Design review of the part built by this model. Coordinates are the model's own, in mm. Face numbers are marked on the shaded views. A direction names the side the tool comes from. Coordinates: 2 decimals unless noted, no trailing zeros. Order: outer loops, then holes, each group sorted by start corner. A loop starts at its lowest first (then second) coordinate and runs counter-clockwise, first axis right, second up. Notation, with made-up numbers: M 73.5,9.25 L 111.5,9.25 A19 ccw 111.5,20.25 Z; hole C 57,59 d4. An arc over 180 degrees is marked long. Answer in a Markdown table with one row per item.
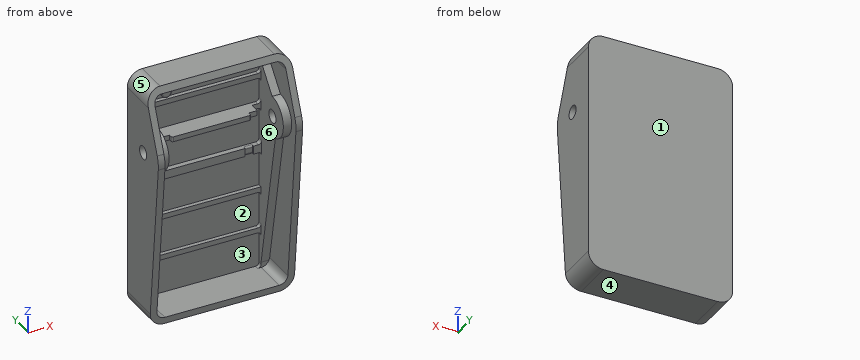
from build123d import *

# Parameters (mm, degrees)
SKETCH4_W           = 86.6
SKETCH4_H           = 145
SKETCH4_W_2         = 78.6
SKETCH4_H_2         = 137
BOSS_EXTRUDE2_DEPTH = 30
SKETCH5_W           = 86.6
SKETCH5_H           = 145
BOSS_EXTRUDE3_DEPTH = 5
SKETCH6_R           = 4
CUT_EXTRUDE2_DEPTH  = 56.5
BOSS_EXTRUDE1_START = 5
SKETCH1_R           = 4
BOSS_EXTRUDE1_DEPTH = 5
SKETCH7_W           = 68.6
SKETCH7_H           = 15.75
SKETCH7_H_2         = 22.125
CUT_EXTRUDE3_DEPTH  = 2.5
FILLET1_R           = 9
SKETCH12_W          = 57.6
SKETCH12_H          = 3
BOSS_EXTRUDE6_DEPTH = 8.5
SKETCH13_W          = 5
SKETCH13_H          = 2.5
CUT_EXTRUDE4_DEPTH  = 5
FILLET6_R           = 1
FILLET2_R           = 2
FILLET3_R           = 5
SKETCH10_R          = 3
BOSS_EXTRUDE4_DEPTH = 2.5
FILLET4_R           = 0.5
SKETCH11_W          = 48.6
SKETCH11_H          = 5
BOSS_EXTRUDE5_DEPTH = 0.75
FILLET5_R           = 1


with BuildPart() as part:
    # Sketch4 → Boss-Extrude2 (new body)
    with BuildSketch(Plane(origin=(0, 12.8, 0), x_dir=(1, 0, 0), z_dir=(0, 1, 0))):
        with Locations((0, 32.5)):
            Rectangle(SKETCH4_W, SKETCH4_H)
        with Locations((0, 32.5)):
            Rectangle(SKETCH4_W_2, SKETCH4_H_2, mode=Mode.SUBTRACT)
    extrude(amount=-BOSS_EXTRUDE2_DEPTH)

    # Sketch5 → Boss-Extrude3 (add)
    with BuildSketch(Plane(origin=(0, 12.8, 0), x_dir=(1, 0, 0), z_dir=(0, 1, 0))):
        with Locations((0, 32.5)):
            Rectangle(SKETCH5_W, SKETCH5_H)
    extrude(amount=BOSS_EXTRUDE3_DEPTH)

    # Sketch6 → Cut-Extrude2 (cut, symmetric)
    with BuildSketch(Plane(origin=(0, 0, 0), x_dir=(0, 0, -1), z_dir=(1, 0, 0))):
        Circle(SKETCH6_R)
        with BuildLine():
            Line((-40, -2.2), (-6.520615654, -15.916079024))
            ThreePointArc((-6.520615654, -15.916079024), (-2.511916424, -17.015589202), (1.643491767, -17.121300617))
            Line((1.643491767, -17.121300617), (105, -7.2))
            Line((105, -7.2), (105, -30))
            Line((105, -30), (-40, -30))
            Line((-40, -30), (-40, -2.2))
        make_face()
    extrude(amount=CUT_EXTRUDE2_DEPTH, both=True, mode=Mode.SUBTRACT)

    # Sketch1 → Boss-Extrude1 (add)
    with BuildSketch(Plane(origin=(-39.3, 0, 0), x_dir=(0, 0, -1), z_dir=(1, 0, 0)).offset(BOSS_EXTRUDE1_START)):
        with BuildLine():
            Line((-12.295827489, 0.320353501), (-27.31993911, 12.8))
            Line((-27.31993911, 12.8), (97.713486421, 12.8))
            Line((97.713486421, 12.8), (11.842309408, -3.324110088))
            ThreePointArc((11.842309408, -3.324110088), (-1.836286572, -12.162156537), (-12.295827489, 0.320353501))
        make_face()
        Circle(SKETCH1_R, mode=Mode.SUBTRACT)
    boss_extrude1 = extrude(amount=-BOSS_EXTRUDE1_DEPTH)

    # Mirror1: Boss-Extrude1 across plane
    add(boss_extrude1.mirror(Plane(origin=(0, 0, 0), x_dir=(0, 0, 1), z_dir=(1, 0, 0))))

    # Sketch7 → Cut-Extrude3 (cut)
    with BuildSketch(Plane.XZ.offset(-12.8)):
        with Locations((0, 28.125)):
            Rectangle(SKETCH7_W, SKETCH7_H)
        with Locations((0, -89.9375)):
            Rectangle(SKETCH7_W, SKETCH7_H_2)
        with Locations((0, 9.375)):
            Rectangle(SKETCH7_W, SKETCH7_H)
        with Locations((0, -12.5625)):
            Rectangle(SKETCH7_W, SKETCH7_H_2)
        with Locations((0, -39.6875)):
            Rectangle(SKETCH7_W, SKETCH7_H_2)
        with Locations((0, -64.8125)):
            Rectangle(SKETCH7_W, SKETCH7_H_2)
    extrude(amount=-CUT_EXTRUDE3_DEPTH, mode=Mode.SUBTRACT)

    # Fillet1
    fillet1_edges = [part.edges().sort_by_distance(p)[0] for p in [
        (43.3, 7.8, 40),
        (-43.3, 7.8, 40),
        (43.3, 5.3, -105),
        (-43.3, 5.3, -105),
    ]]
    fillet(fillet1_edges, radius=FILLET1_R)

    # Sketch12 → Boss-Extrude6 (add)
    with BuildSketch(Plane.XZ.offset(-12.8)):
        Rectangle(SKETCH12_W, SKETCH12_H)
    extrude(amount=BOSS_EXTRUDE6_DEPTH)

    # Sketch13 → Cut-Extrude4 (cut)
    with BuildSketch(Plane(origin=(0, 0, -1.5), x_dir=(-1, 0, 0), z_dir=(0, 0, -1))):
        with Locations((-26.3, 5.55)):
            Rectangle(SKETCH13_W, SKETCH13_H)
        with Locations((26.3, 5.55)):
            Rectangle(SKETCH13_W, SKETCH13_H)
    extrude(amount=-CUT_EXTRUDE4_DEPTH, mode=Mode.SUBTRACT)

    # Fillet6
    fillet6_edges = [part.edges().sort_by_distance(p)[0] for p in [
        (-23.8, 4.3, 0),
        (23.8, 4.3, 0),
    ]]
    fillet(fillet6_edges, radius=FILLET6_R)

    # Fillet2
    fillet2_edges = [part.edges().sort_by_distance(p)[0] for p in [
        (-34.3, 14.05, 20.25),
        (-34.3, 14.05, 36),
        (34.3, 14.05, 36),
        (34.3, 14.05, 20.25),
        (-34.3, 14.05, -75.875),
        (-34.3, 14.05, -53.75),
        (34.3, 14.05, -53.75),
        (34.3, 14.05, -75.875),
        (34.3, 14.05, -78.875),
        (34.3, 14.05, -101),
        (-34.3, 14.05, -101),
        (-34.3, 14.05, -78.875),
        (-34.3, 14.05, 1.5),
        (-34.3, 14.05, 17.25),
        (34.3, 14.05, 17.25),
        (34.3, 14.05, 1.5),
        (-34.3, 14.05, -23.625),
        (-34.3, 14.05, -1.5),
        (34.3, 14.05, -1.5),
        (34.3, 14.05, -23.625),
        (-34.3, 14.05, -50.75),
        (-34.3, 14.05, -28.625),
        (34.3, 14.05, -28.625),
    ]]
    fillet(fillet2_edges, radius=FILLET2_R)

    # Fillet3
    fillet3_edges = [part.edges().sort_by_distance(p)[0] for p in [
        (39.3, 4.480625373, 36),
        (-39.3, 4.480625373, 36),
        (39.3, 2.608017883, -101),
        (-39.3, 2.608017883, -101),
    ]]
    fillet(fillet3_edges, radius=FILLET3_R)

    # Sketch10 → Boss-Extrude4 (add)
    with BuildSketch(Plane.XZ.offset(-15.3)):
        with Locations(Location((-22.3, 24, 0), (0, 0, 270))):
            Circle(SKETCH10_R)
    extrude(amount=BOSS_EXTRUDE4_DEPTH)

    # Fillet4
    fillet4_edges = [part.edges().sort_by_distance(p)[0] for p in [
        (-22.3, 12.8, 27),
    ]]
    fillet(fillet4_edges, radius=FILLET4_R)

    # Sketch11 → Boss-Extrude5 (add, symmetric)
    with BuildSketch(Plane.XZ.offset(-12.8)):
        with BuildLine():
            Line((-29.3, -23.625), (-32.3, -23.625))
            ThreePointArc((-32.3, -23.625), (-33.714213562, -23.039213562), (-34.3, -21.625))
            Line((-34.3, -21.625), (-34.3, -30.625))
            ThreePointArc((-34.3, -30.625), (-33.714213562, -29.210786438), (-32.3, -28.625))
            Line((-32.3, -28.625), (-29.3, -28.625))
            Line((-29.3, -28.625), (-29.3, -23.625))
        make_face()
        with BuildLine():
            Line((32.3, -23.625), (29.3, -23.625))
            Line((29.3, -23.625), (29.3, -28.625))
            Line((29.3, -28.625), (32.3, -28.625))
            ThreePointArc((32.3, -28.625), (33.714213562, -29.210786438), (34.3, -30.625))
            Line((34.3, -30.625), (34.3, -21.625))
            ThreePointArc((34.3, -21.625), (33.714213562, -23.039213562), (32.3, -23.625))
        make_face()
        with Locations((0, -26.125)):
            Rectangle(SKETCH11_W, SKETCH11_H)
    extrude(amount=BOSS_EXTRUDE5_DEPTH, both=True)

    # Fillet5
    fillet5_edges = [part.edges().sort_by_distance(p)[0] for p in [
        (26.8, 12.8, -28.625),
        (-26.8, 12.8, -23.625),
        (26.8, 12.8, -23.625),
        (-26.8, 12.8, -28.625),
    ]]
    fillet(fillet5_edges, radius=FILLET5_R)


solid = part.part
(1) Add section B-B, the plane x = -10.5. Give the boundary of the cut face in (y, z) (3 decimals), and give its area (3 significant figures).
Return value:
| item | result |
|---|---|
| outline | M -7.584,-101 L -7.2,-105 L 17.8,-105 L 17.8,40 L -2.2,40 L -3.839,36 L 15.3,36 L 15.3,20.25 L 12.8,20.25 L 12.8,17.25 L 15.3,17.25 L 15.3,1.5 L 4.3,1.5 L 4.3,-1.5 L 15.3,-1.5 L 15.3,-23.625 L 12.05,-23.625 L 12.05,-28.625 L 15.3,-28.625 L 15.3,-50.75 L 12.8,-50.75 L 12.8,-53.75 L 15.3,-53.75 L 15.3,-75.875 L 12.8,-75.875 L 12.8,-78.875 L 15.3,-78.875 L 15.3,-101 Z |
| area | 598 mm2 |
(2) For the marked faces 5 and 6, list the 3-axis set-ups (+Z, -Z, +X, -X, +Y, -Y) from which the entire face can be reached by the end or side of a thin tool; tool diameter is ignored.
Return value:
| item | result |
|---|---|
| face 5 | +Z, -X, +Y, -Y |
| face 6 | -Y |
(3) Add section A-A, the plane z = 0. Give the number of separate pieces and of enclosed holes in the cut face, and give its area (3 significant figures).
Return value:
| item | result |
|---|---|
| separate pieces | 3 |
| enclosed holes | 0 |
| area | 1,240 mm2 |
(4) Add section C-C, the plane z = 24. Give the boundary of the cut face in (x, y) (3 decimals), and give its area (3 significant figures).
Return value:
| item | result |
|---|---|
| outline | M -43.3,-8.755 L -39.3,-8.755 L -39.3,10.042 L -34.3,10.042 L -34.3,15.3 L -25.3,15.3 L -25.3,13.3 A0.5 ccw -24.8,12.8 L -19.8,12.8 A0.5 ccw -19.3,13.3 L -19.3,15.3 L 34.3,15.3 L 34.3,10.042 L 39.3,10.042 L 39.3,-8.755 L 43.3,-8.755 L 43.3,17.8 L -43.3,17.8 Z |
| area | 476 mm2 |
(5) Insertion check: pin 1 Ø1.5 at (x, z) = (5, -27) entering from -Y; pin 2 Ø9 at (y, z) = (0, 0) entering from +X; pin 3 Ø1.5 at (x, z) = (-4, 3) entering from -Y; pin 4 Ø7.5 at (x, z) = (0.5, 17) entering from -Y. Each pin has a flat end and moves straight along its axis. Give the tip position at first contact, or say it passes through.
Return value:
| item | result |
|---|---|
| pin 1 | stops at y = 12.05 |
| pin 2 | stops at x = 43.3 |
| pin 3 | stops at y = 15.3 |
| pin 4 | stops at y = 12.8 |
(6) Add section D-D, the plane z = -18.5. Give the boundary of the cut face in (x, y), and give its area (3 significant figures).
Return value:
| item | result |
|---|---|
| outline | M -43.3,-15.5 L -39.3,-15.5 L -39.3,-2.07 L -34.3,-2.07 L -34.3,15.3 L 34.3,15.3 L 34.3,-2.07 L 39.3,-2.07 L 39.3,-15.5 L 43.3,-15.5 L 43.3,17.8 L -43.3,17.8 Z |
| area | 637 mm2 |
(7) Draft analysis for pull direction Z (two halves, no side actions). For the marked faces 1, 2, 3 and 4, state which applies: pulls with the +Z half, pulls with the -Z half, needs draft (parallel to the pull), parting line crosses it, or undercut.
Return value:
| item | result |
|---|---|
| face 1 | needs draft |
| face 2 | undercut |
| face 3 | undercut |
| face 4 | pulls with the -Z half |
(8) For line 1 along Z through (x, y) = (17, 7); line 2 along Y through (x, z) = (39.5, 0); line 3 along X through (y, z) = (-8.5, -83), list the stretches that pass through material, from the lowest coordinate up. Write a range as from..to.
Return value:
| item | result |
|---|---|
| line 1 | z = -105..-101, -1.5..1.5, 36..40 |
| line 2 | y = -17.2..-4, 4..17.8 |
| line 3 | x = -43.3..-39.3, 39.3..43.3 |
